Build history of the part. All positions in model axes, mm. Give positions to 0.01 mm unless a question says otherwise; leave off trailing zeros. Loops run counter-clockwise (first coordinate to the right, second up) from the corner with the lowest first, then second, coordinate; pieces in that order, holes last. Notation, with made-up numbers: (71.5, -39) -> (119.5, -39) arc R19 cw to (119.5, -16) -> close; hole circle Ø4 at (32.5, 40). An arc over 180 degrees is marked (long way). Answer as a JSON object with one key per item and string values. Group by question number.
Q1. Band-saw the part on C-C, the plane x = 14. Write the cut outline in (y, z).
Q2. Band-saw the part on D-D, the plane z = 17.5. Write the cut outline in (x, y).
Q3. Wall check: probe 1 along Y at (x, z) = (16.5, 6); probe 2 along Y at (x, z) = (15.5, -5.5); probe 3 along Z at (x, y) = (6.75, 0). Give the ranges that are in metal, low to high. Write a range as from..to.
Q4. Band-saw the part on A-A, the plane y = 0. Write the cut outline in (x, z), plus the area to 3 significant figures.
Q5. Drop flat-ended pins along their axis: pin 1 (1 mm diameter, centred on x = 8, y = -18, fed in from -Z); pin 2 (2 mm diameter, centred on x = 13.5, y = -20, fed in from +Z); pin 3 (4 mm diameter, centred on x = 5, z = 6.5, fed in from +Y). Give the stop position or say it passes through.
Autodesk Inventor part; units mm, degrees
ref_plane "YZ Plane" through (0, 0, 0) normal (1, 0, 0) x (0, 1, 0)
ref_plane "XZ Plane" through (0, 0, 0) normal (0, 1, 0) x (-1, 0, 0)
ref_plane "XY Plane" through (0, 0, 0) normal (0, 0, 1) x (1, 0, 0)
sketch "Sketch1" plane through (0, 0, 0) normal (1, 0, 0) x (0, 1, 0)
  circle A0 centre (0, 0) radius 27
  circle A1 centre (0, 0) radius 8 construction
  line L0 (-8, 8) -> (8, 8) construction
  line L1 (8, 8) -> (8, -8) construction
  line L2 (8, -8) -> (-8, -8) construction
  line L3 (-8, -8) -> (-8, 8) construction
  line L4 (-8, 8) -> (8, -8) construction
  line L5 (8, 8) -> (-8, -8) construction
  circle A2 centre (5.6569, 5.6569) radius 1.6
  circle A3 centre (5.6569, -5.6569) radius 1.5
  circle A4 centre (-5.6569, -5.6569) radius 1.6
  circle A5 centre (-5.6569, 5.6569) radius 1.5
  circle A6 centre (0, 0) radius 3
  dimension "d0" = 54
  dimension "d1" = 16
  dimension "d2" = 3.2
  dimension "d3" = 3
  dimension "d4" = 3.2
  dimension "d5" = 3
  dimension "d6" = 6
  dimension "d7" = 16
  dimension "d8" = 16
extrude "Extrusion1" add sketch "Sketch1" along normal blind 25.4
properties part number "60mm_Grip_Wheel"
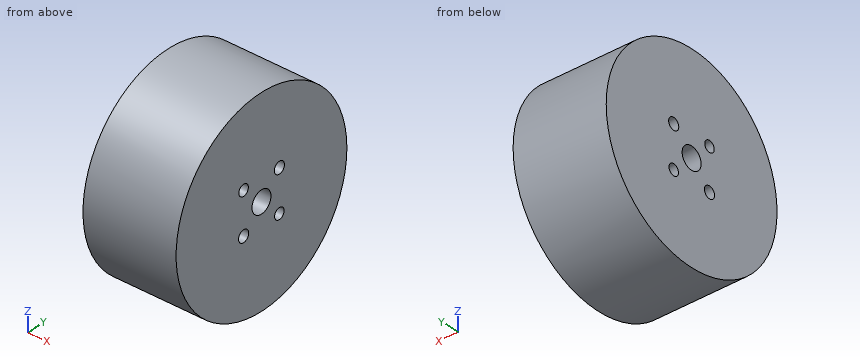
Worked answers:
{
 "1": {"outline": "circle Ø54 at (0, 0); hole circle Ø3.2 at (-5.66, -5.66); hole circle Ø3 at (-5.66, 5.66); hole circle Ø6 at (0, 0); hole circle Ø3.2 at (5.66, 5.66); hole circle Ø3 at (5.66, -5.66)"},
 "2": {"outline": "(0, -20.56) -> (25.4, -20.56) -> (25.4, 20.56) -> (0, 20.56) -> close"},
 "3": {"probe 1": "-26.32..-7.12, -4.2..4.09, 7.22..26.32", "probe 2": "-26.43..-7.25, -4.06..4.17, 7.15..26.43", "probe 3": "-27..-3, 3..27"},
 "4": {"outline": "(0, -27) -> (25.4, -27) -> (25.4, -3) -> (0, -3) -> close; (0, 3) -> (25.4, 3) -> (25.4, 27) -> (0, 27) -> close", "area": "1,220 mm2"},
 "5": {"pin 1": "z = -20.56", "pin 2": "z = 19.18", "pin 3": "y = 26.62"}
}
